Read the model definition and answer for the solid it produces. Units are mm, in the model's axes. A direction names the side the tool comes from. Round coordinates to 2 decimals unless told otherwise and drop trailing zeros. Order: outer loops, then holes, each group sorted by start corner. A loop starts at its lowest first (then second) coordinate and runs counter-clockwise, first axis right, second up.
from build123d import *

# Parameters (mm, degrees)
F0_W           = 35.56
F0_H           = 76.2
F1_DEPTH       = 38.1
F3_D           = 9.525
F3_CSINK_D     = 13.4874
F3_CSINK_ANGLE = 82


# Not quite as in the source:
# - a length typed as a fraction of an inch, garbled in the dataset ("3 / 203.2 mm" for 3/8 in), is restored


with BuildPart() as f1:
    # F0 (on Top) → F1 (new body)
    with BuildSketch(Plane.XY):
        with BuildLine():
            Line((97.53417238, 58.7352159441), (-80.26582762, 58.7352159441))
            ThreePointArc((-80.26582762, 58.7352159441), (-89.2460837411, 55.0154720651), (-92.96582762, 46.0352159441))
            Line((-92.96582762, 46.0352159441), (-92.96582762, 33.3352159441))
            Line((-92.96582762, 33.3352159441), (-57.40582762, 33.3352159441))
            Line((-57.40582762, 33.3352159441), (74.67417238, 33.3352159441))
            Line((74.67417238, 33.3352159441), (110.23417238, 33.3352159441))
            Line((110.23417238, 33.3352159441), (110.23417238, 46.0352159441))
            ThreePointArc((110.23417238, 46.0352159441), (106.514428501, 55.0154720651), (97.53417238, 58.7352159441))
        make_face()
        with Locations((-75.18582762, -4.7647840559)):
            Rectangle(F0_W, F0_H)
        with Locations((92.45417238, -4.7647840559)):
            Rectangle(F0_W, F0_H)
    extrude(amount=F1_DEPTH)

    # F3 (through all)
    with Locations(Plane.XY.offset(38.1)):
        with Locations((-75.50332762, -19.0544008167), (92.77167238, -19.0544008167)):
            CounterSinkHole(F3_D / 2, F3_CSINK_D / 2, counter_sink_angle=F3_CSINK_ANGLE)


solid = f1.part
Q1. Flat-ended cylindrical pins translate along their axes: pin 1 (1 mm diameter, centred on x = 56.5, z = 34, fed in from -Y); pin 2 (11 mm diameter, centred on x = -75.5, y = -19.05, fed in from +Z). Find the tip coordinate at first contact, or state that the pin passes through.
Outcome:
pin 1: stops at y = 33.34
pin 2: stops at z = 36.68
Q2. Straight lines are drawn through the part: probe 1 along X at (y, z) = (25, 23.5); probe 2 along X at (y, z) = (-22, 32); probe 3 along Y at (x, z) = (89, 30). For each, find the intervals that lie inside material, in ascending order.
Outcome:
probe 1: x = -92.97 to -57.41, 74.67 to 110.23
probe 2: x = -92.97 to -79.25, -71.76 to -57.41, 74.67 to 89.03, 96.51 to 110.23
probe 3: y = -42.86 to -21.96, -16.15 to 58.74
Q3. A cutting plane is placed at B-B, the plane z = 32. Give the vertices of the cut face in (x, y) (1 decimal), plus the area to 3 significant figures.
Outcome:
outline: (-93, -42.9) - (-57.4, -42.9) - (-57.4, 33.3) - (74.7, 33.3) - (74.7, -42.9) - (110.2, -42.9) - (110.2, 46) arc R12.7 ccw to (97.5, 58.7) - (-80.3, 58.7) arc R12.7 ccw to (-93, 46) - close; hole circle Ø9.5 at (-75.5, -19.1); hole circle Ø9.5 at (92.8, -19.1)
area: 10,400 mm2
Q4. For a pull along Y with two mould halves and no side action, classify faces 1 (the face through (-70.745, -18.845, 17.66)), 2 (the face through (7, 43, 0)), 3 (the face through (88.372, -20.878, 17.66)), 4 (the face through (-75, -42.865, 19)) as released by +Y, released by -Y, zero draft, split by the parting line, or undercut.
Outcome:
face 1: undercut
face 2: zero draft
face 3: undercut
face 4: released by -Y
Q5. A cutting plane is placed at A-A, the plane y = -30. Give the vertices of the cut face in (x, z), plus the area to 3 significant figures.
Outcome:
outline: (-92.97, 0) - (-57.41, 0) - (-57.41, 38.1) - (-92.97, 38.1) - close; (74.67, 0) - (110.23, 0) - (110.23, 38.1) - (74.67, 38.1) - close
area: 2,710 mm2
Q6. For faces 5 (the face through (10, 58.735, 19)), 6 (the face through (-57.406, -5, 19)), determine the directions among +Z, -Z, +X, -X, +Y, -Y from which every point of the face is accessible in a straight line to the end or side of a thin tool.
Outcome:
face 5: +Z, -Z, +X, -X, +Y
face 6: +Z, -Z, -Y
Q7. A cutting plane is placed at C-C, the plane x = 30. Give the vertices of the cut face in (y, z).
Outcome:
outline: (33.34, 0) - (58.74, 0) - (58.74, 38.1) - (33.34, 38.1) - close
